Design review of the part built by this model. Coordinates are the model's own, in mm. Coordinates: 2 decimals unless noted, no trailing zeros. Write each loop counter-clockwise with the first axis right and the second up, starting at its lowest first coordinate (ties: lowest second). Pieces come first, ordered by that corner, then holes.
Q1. Clearance check with flat-ended pins moving along their axes: pin 1 Ø0.9 at (y, z) = (26.5, 2) entering from -X; pin 2 Ø0.9 at (y, z) = (-10.5, 1) entering from -X; pin 3 Ø1.5 at (y, z) = (-26.5, 2) entering from +X. State where each tip first meets the part, or that it passes through.
Q2. To check wall thickness, follow probe 1 along X at (y, z) = (-14.5, 0.5); probe 2 along X at (y, z) = (-25.5, 1.15); probe 3 along X at (y, z) = (19, 2.55). State the ranges of each line that lie inside material, in increasing order.
Q3. Add section A-A, the plane x = 122.5. Give the boundary of the cut face in (y, z), plus the area to 3 significant figures.
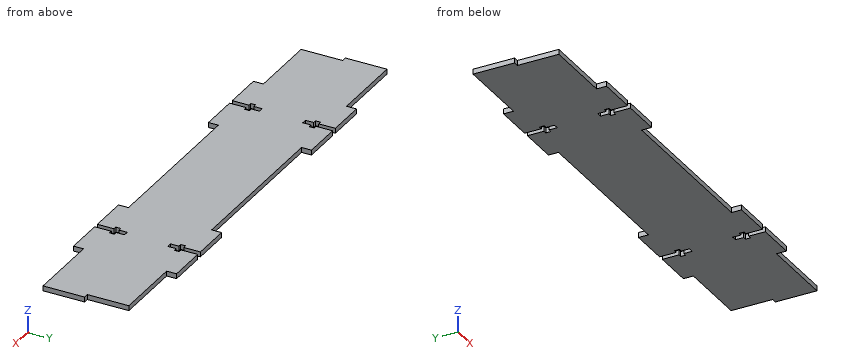
from build123d import *

# Parameters (mm, degrees)
BOSS_EXTRUDE1_DEPTH = 3
CUT_EXTRUDE1_DEPTH  = 10


with BuildPart() as part:
    # Sketch1 → Boss-Extrude1 (new body)
    with BuildSketch(Plane.XY):
        Polygon((-145, 0), (-142, 0), (-142, -25), (-100, -25), (-100, -31), (-50, -31), (-50, -25), (50, -25), (50, -31), (100, -31), (100, -25), (145, -25), (145, 0), (142, 0), (142, 25), (100, 25), (100, 31), (50, 31), (50, 25), (-50, 25), (-50, 31), (-100, 31), (-100, 25), (-145, 25), align=None)
    extrude(amount=BOSS_EXTRUDE1_DEPTH)

    # Sketch2 → Cut-Extrude1 (cut)
    with BuildSketch(Plane.XY.offset(3)):
        Polygon((-75, 31), (-76.5, 31), (-76.5, 21), (-78.5, 21), (-78.5, 18), (-76.5, 18), (-76.5, 13), (-73.5, 13), (-73.5, 18), (-71.5, 18), (-71.5, 21), (-73.5, 21), (-73.5, 31), align=None)
        Polygon((-76.5, -31), (-76.5, -21), (-78.5, -21), (-78.5, -18), (-76.5, -18), (-76.5, -13), (-73.5, -13), (-73.5, -18), (-71.5, -18), (-71.5, -21), (-73.5, -21), (-73.5, -31), align=None)
        Polygon((73.5, 31), (73.5, 21), (71.5, 21), (71.5, 18), (73.5, 18), (73.5, 13), (76.5, 13), (76.5, 18), (78.5, 18), (78.5, 21), (76.5, 21), (76.5, 31), align=None)
        Polygon((73.5, -31), (73.5, -21), (71.5, -21), (71.5, -18), (73.5, -18), (73.5, -13), (76.5, -13), (76.5, -18), (78.5, -18), (78.5, -21), (76.5, -21), (76.5, -31), align=None)
    extrude(amount=-CUT_EXTRUDE1_DEPTH, mode=Mode.SUBTRACT)


solid = part.part
Here are the results:
1. pin 1: stops at x = -100
1. pin 2: stops at x = -142
1. pin 3: stops at x = 100
2. probe 1: x = -142 to -76.5, -73.5 to 73.5, 76.5 to 145
2. probe 2: x = -100 to -76.5, -73.5 to -50, 50 to 73.5, 76.5 to 100
2. probe 3: x = -145 to -78.5, -71.5 to 71.5, 78.5 to 142
3. outline: (-25, 0) - (25, 0) - (25, 3) - (-25, 3) - close
3. area: 150 mm2
